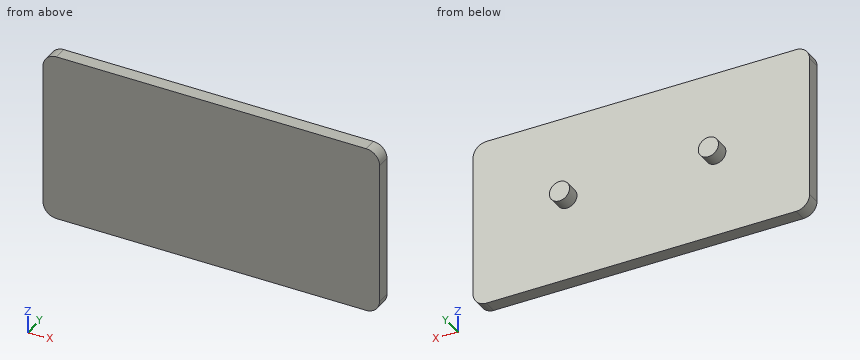
```python
from build123d import *

# Parameters (mm, degrees)
SKETCH1_W           = 635
SKETCH1_H           = 317.5
BOSS_EXTRUDE1_DEPTH = 25.4
SKETCH2_R           = 19.05
BOSS_EXTRUDE2_DEPTH = 25.4
FILLET1_R           = 25.4


with BuildPart() as part:
    # Sketch1 → Boss-Extrude1 (new body)
    with BuildSketch(Plane(origin=(0, 0, 0), x_dir=(1, 0, 0), z_dir=(0, 1, 0))):
        Rectangle(SKETCH1_W, SKETCH1_H)
    extrude(amount=BOSS_EXTRUDE1_DEPTH)

    # Sketch2 → Boss-Extrude2 (add)
    with BuildSketch(Plane(origin=(0, 25.4, 0), x_dir=(1, 0, 0), z_dir=(0, 1, 0))):
        with Locations(Location((-140.462, 0, 0), (0, 0, 270))):
            Circle(SKETCH2_R)
        with Locations(Location((140.462, 0, 0), (0, 0, 90))):
            Circle(SKETCH2_R)
    extrude(amount=BOSS_EXTRUDE2_DEPTH)

    # Fillet1
    fillet1_edges = [part.edges().sort_by_distance(p)[0] for p in [
        (317.5, 12.7, 158.75),
        (-317.5, 12.7, 158.75),
        (-317.5, 12.7, -158.75),
        (317.5, 12.7, -158.75),
    ]]
    fillet(fillet1_edges, radius=FILLET1_R)


solid = part.part
```
Geometry check sheet. Reference: the model listing, model coordinates, mm. Give positions to 0.01 mm unless a question says otherwise; leave off trailing zeros. Write each loop counter-clockwise with the first axis right and the second up, starting at its lowest first coordinate (ties: lowest second). Pieces come first, ordered by that corner, then holes.
1) Section check D-D, the plane z = 114. Record the boundary of the cut face in (x, y), and give its area (3 significant figures).
2) Gauge pin test, flat end, axial feed: pin 1 (2 mm diameter, centred on x = -15, y = 28, fed in from +Z). Record the tip position at first contact, or that the pin passes through.
3) Section check C-C, the plane y = 45. Record the boundary of the cut face in (x, z).
4) Section check B-B, the plane x = 106.5. Record the boundary of the cut face in (y, z).
5) Material ranges on L1, parallel to Y at x = 196.5, z = 51.5; L2, parallel to Z at x = 146, y = 47.5; L3, parallel to Z at x = -138, y = 47, recorded low to high.
6) Section check A-A, the plane z = 0. Record the boundary of the cut face in (x, y), and give its area (3 significant figures).
Computed:
1. outline: (-317.5, 0) - (317.5, 0) - (317.5, 25.4) - (-317.5, 25.4) - close
1. area: 16,100 mm2
2. pin 1: passes through
3. outline: circle Ø38.1 at (-140.46, 0); circle Ø38.1 at (140.46, 0)
4. outline: (0, -158.75) - (25.4, -158.75) - (25.4, 158.75) - (0, 158.75) - close
5. L1: y = 0 to 25.4
5. L2: z = -18.23 to 18.23
5. L3: z = -18.89 to 18.89
6. outline: (-317.5, 0) - (317.5, 0) - (317.5, 25.4) - (159.51, 25.4) - (159.51, 50.8) - (121.41, 50.8) - (121.41, 25.4) - (-121.41, 25.4) - (-121.41, 50.8) - (-159.51, 50.8) - (-159.51, 25.4) - (-317.5, 25.4) - close
6. area: 18,100 mm2
